Autodesk Inventor part; units mm, degrees
ref_plane "YZ Plane" through (0, 0, 0) normal (1, 0, 0) x (0, 1, 0)
ref_plane "XZ Plane" through (0, 0, 0) normal (0, 1, 0) x (-1, 0, 0)
ref_plane "XY Plane" through (0, 0, 0) normal (0, 0, 1) x (1, 0, 0)
sketch "Sketch1" plane through (0, 0, 0) normal (0, 1, 0) x (-1, 0, 0)
  line L0 (0.53, 20.25) -> (-28.77, 20.25)
  line L1 (-28.77, 20.25) -> (-28.77, -20.25)
  line L2 (-28.77, -20.25) -> (0.53, -20.25)
  line L3 (0.53, -20.25) -> (0.53, 20.25)
  point P0 (0, 0)
  dimension "d0" = 40.5
  dimension "d1" = 29.3
  dimension "d2" = -0.53
  dimension "d3" = 20.25
extrude "Plate1" add sketch "Sketch1" along normal blind 1.5
sketch "Sketch2" plane through (28.77, 0, 21.75) normal (0, 0, -1) x (-1, 0, 0)
  line L0 (29.3, 0) -> (0, 0)
  line L1 (0, 0) -> (0, 28.14)
  line L2 (0, 28.14) -> (29.3, 28.14)
  line L3 (29.3, 28.14) -> (29.3, 0)
edge flange "Flange1" height 28.14 angle 90 thickness 1.5 bend radius 0.31 thickness toward (0, 0, -1) relief tear relief width 1.5 relief depth 0.75 corner gap 0.31 corner form 0 edges at (14.12, 1.5, 20.25) (14.12, 1.5, -20.25) wall of the first edge with corners at (-0.53, 0, 21.75) (28.77, 0, 21.75) (28.77, 28.14, 21.75) (-0.53, 28.14, 21.75)
bend "Bend1"
corner "Corner1"
sketch "Sketch6" plane through (-0.53, 28.14, 21.75) normal (0, 0, 1) x (1, 0, 0)
  point P0 (0.53, -28.14)
sketch "Sketch8" plane through (28.77, 28.14, -21.75) normal (0, 0, -1) x (-1, 0, 0)
  circle A0 centre (2.5, -2.545) radius 0.7835
  circle A1 centre (2.5, -17.595) radius 0.7835
  circle A2 centre (17.6, -2.545) radius 0.7835
  circle A3 centre (17.6, -17.595) radius 0.7835
  circle A4 centre (37.6, -2.545) radius 0.7835
  circle A5 centre (37.6, -17.595) radius 0.7835
  point P0 (28.77, -28.14)
hole "Hole4" at (26.27, 25.595, -21.75) at (26.27, 10.545, -21.75) at (11.17, 25.595, -21.75) at (11.17, 10.545, -21.75) at (-8.83, 25.595, -21.75) at (-8.83, 10.545, -21.75) direction (0, 0, 1) diameter 2.1 depth 1.5
sketch "Sketch9" plane through (28.77, 28.14, -21.75) normal (0, 0, -1) x (-1, 0, 0)
  circle A0 centre (30.1, -10.07) radius 6
  point P0 (28.77, -28.14)
extrude "Cut2" cut sketch "Sketch9" against normal blind 1.5
sketch "Sketch10" plane through (-0.53, 28.14, 21.75) normal (0, 0, 1) x (1, 0, 0)
  point P0 (0.53, -28.14)
sketch "Sketch11" plane through (-0.53, 28.14, 21.75) normal (0, 0, 1) x (1, 0, 0)
  point P0 (0.53, -28.14)
sketch "Sketch15" plane through (0, 0, 0) normal (0, -1, 0) x (1, 0, 0)
  point P0 (0, 0)
sketch "Sketch16" plane through (0, 0, 0) normal (0, -1, 0) x (1, 0, 0)
  circle A0 centre (6.47, 14.94) radius 1.55
  line L0 (28.77, 19.94) -> (-0.53, 19.94)
  line L1 (-0.53, -19.94) -> (-0.53, 19.94)
  circle A1 centre (21.77, 14.94) radius 1.55
  line L2 (28.77, 19.94) -> (28.77, -19.94)
  circle A2 centre (6.47, 4.8) radius 1.55
  circle A3 centre (21.77, 4.8) radius 1.55
  point P0 (0, 0)
  dimension "d65" = 3.1
  dimension "d66" = 5
  dimension "d67" = 7
  dimension "d68" = 3.1
  dimension "d69" = 5
  dimension "d70" = 7
  dimension "d71" = 3.1
  dimension "d72" = 15.14
  dimension "d73" = 7
  dimension "d74" = 3.1
  dimension "d75" = 15.14
  dimension "d76" = 7
extrude "Cut6" cut sketch "Sketch16" against normal blind 1.5
sketch "Sketch18" plane through (-0.53, 28.14, 21.75) normal (0, 0, 1) x (1, 0, 0)
  circle A0 centre (-0.8, -10.07) radius 6
  point P0 (0.53, -28.14)
extrude "Cut7" cut sketch "Sketch18" against normal blind 1.5
fillet "Corner Round1" radius 1 4 edges at (-0.53, 28.14, -21) (28.77, 28.14, -21) (28.77, 28.14, 21) (-0.53, 28.14, 21)
sketch "Sketch19" plane through (-0.53, 1.81, 21.75) normal (0, 0, 1) x (1, 0, 0)
  circle A0 centre (6.1, 24.26) radius 0.7835
  circle A1 centre (19.32, 23.26) radius 0.7835
  circle A2 centre (26.62, 16.26) radius 0.7835
  circle A3 centre (19.32, 9.26) radius 0.7835
  circle A4 centre (6.1, 8.26) radius 0.7835
  point P0 (0.53, -1.81)
hole "Hole6" at (5.57, 26.07, 21.75) at (18.79, 25.07, 21.75) at (26.09, 18.07, 21.75) at (18.79, 11.07, 21.75) at (5.57, 10.07, 21.75) direction (0, 0, -1) diameter 2.1 depth 1.5
equation "\"d55\" = Thickness"
equation "\"d57\" = Thickness"
equation "\"d77\" = Thickness"
equation "\"d86\" = Thickness"
equation "\"d94\" = Thickness"
equation "\"d4\" = Thickness"
equation "\"d5\" = BendReliefWidth"
equation "\"d6\" = BendReliefDepth"
equation "\"d7\" = MinimumRemnant"
equation "\"d8\" = TransitionRadius"
equation "\"d11\" = BendRadius"
equation "\"d12\" = CornerReliefSize"
equation "\"d13\" = GapSize"
equation "\"d14\" = JacobiRadiusSize"
equation "\"BendReliefWidth\" = Thickness"
equation "\"BendReliefDepth\" = 0.5 * Thickness"
equation "\"CornerReliefSize\" = 4 * Thickness"
equation "\"MinimumRemnant\" = 2 * Thickness"
equation "\"TransitionRadius\" = BendRadius"
equation "\"JacobiRadiusSize\" = BendRadius"
equation "\"GapSize\" = Thickness"
properties part number "axis_25_bottom_frame" material "Aluminum 6061-AHC"
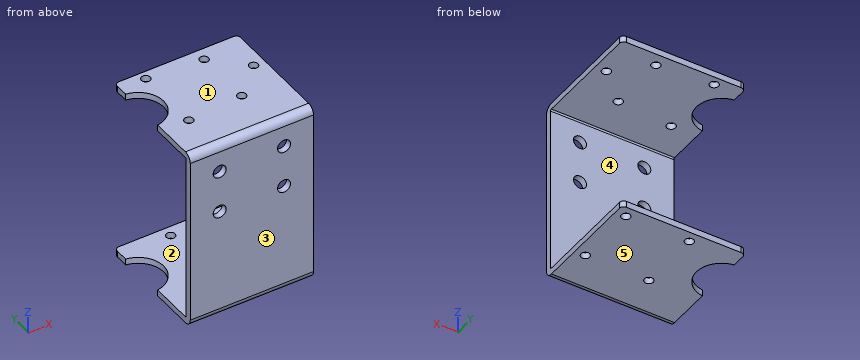
Work out the finished part from the listing and answer in its coordinate system (mm). Face numbers are marked on the shaded views. A direction names the side the tool comes from. Give positions to 0.01 mm unless a question says otherwise; leave off trailing zeros. Write each loop counter-clockwise with the first axis right and the second up, starting at its lowest first coordinate (ties: lowest second). Pieces come first, ordered by that corner, then holes. Notation, with made-up numbers: M 5,32.5 L 30,32.5 A19 cw 30,38.5 Z; hole C 30.5,75.25 d10. An arc over 180 degrees is marked long. Answer as CSV lines item,"result".
Q1. Given P1, Ø14.5, axis at x = 19.5, z = 6.5, coming from the +Y side; P2, Ø1.3, axis at x = 26.09, y = 18.07, coming from the +Z side, each flat-ended and moving along its own axis, determine where each tip first touches the part or whether it passes through.
A:
P1,"stops at y = 1.5"
P2,"stops at z = -20.25"
Q2. The mould has two halves that part along Z. Classify the marked faces 3, 4 and 5: +Z half, -Z half, draft (parallel to the pull), parting line (faces both ways), or undercut.
A:
face 3,"draft"
face 4,"undercut"
face 5,"-Z half"
Q3. A tool of negligible diameter and unlimited length cuts with its end or side. For the marked faces 1 and 2, from which of +Z, -Z, +X, -X, +Y, -Y can it reach the whole face along a straight path? Write none if from no direction.
A:
face 1,"+Z, +X, -X, +Y, -Y"
face 2,"+X, -X, +Y"
Q4. Find the intervals of material crossed by probe 1 along Y at (x, z) = (18.79, 21.15); probe 2 along Z at (x, y) = (17.75, 13.5); probe 3 along Z at (x, y) = (6.47, 0.55), in increasing order. Write a range as [from, to].
A:
probe 1,"y = [0.46, 10.02], [12.12, 24.02], [26.12, 28.14]"
probe 2,"z = [-21.75, -20.25], [20.25, 21.75]"
probe 3,"z = [-21.24, 3.25], [6.35, 13.39], [16.49, 21.24]"
Q5. A cutting plane is placed at C-C on y = 6.5. Write down the section's boundary in (x, z).
A:
outline,"M -0.53,-21.75 L 28.77,-21.75 L 28.77,-20.25 L -0.53,-20.25 Z; M -0.53,20.25 L 28.77,20.25 L 28.77,21.75 L -0.53,21.75 Z"
Q6. A cutting plane is placed at A-A on x = 18.79. Write down the section's boundary in (y, z), plus the area to 3 significant figures.
A:
outline,"M 0,-19.94 A1.81 ccw 1.81,-21.75 L 28.14,-21.75 L 28.14,-20.25 L 1.81,-20.25 A0.31 cw 1.5,-19.94 L 1.5,19.94 A0.31 cw 1.81,20.25 L 10.02,20.25 L 10.02,21.75 L 1.81,21.75 A1.81 ccw 0,19.94 Z; M 12.12,20.25 L 24.02,20.25 L 24.02,21.75 L 12.12,21.75 Z; M 26.12,20.25 L 28.14,20.25 L 28.14,21.75 L 26.12,21.75 Z"
area,"138 mm²"
Q7. A cutting plane is placed at B-B on z = 4.8. Write down the section's boundary in (x, y).
A:
outline,"M -0.53,0 L 4.92,0 L 4.92,1.5 L -0.53,1.5 Z; M 8.02,0 L 20.22,0 L 20.22,1.5 L 8.02,1.5 Z; M 23.32,0 L 28.77,0 L 28.77,1.5 L 23.32,1.5 Z"
Q8. A cutting plane is placed at D-D on x = 5.57. Write down the section's boundary in (y, z), plus the area to 3 significant figures.
A:
outline,"M 0,-19.94 A1.81 ccw 1.81,-21.75 L 28.14,-21.75 L 28.14,-20.25 L 1.81,-20.25 A0.31 cw 1.5,-19.94 L 1.5,3.54 L 0,3.54 Z; M 0,6.06 L 1.5,6.06 L 1.5,13.68 L 0,13.68 Z; M 0,16.2 L 1.5,16.2 L 1.5,19.94 A0.31 cw 1.81,20.25 L 9.02,20.25 L 9.02,21.75 L 1.81,21.75 A1.81 ccw 0,19.94 Z; M 11.12,20.25 L 25.02,20.25 L 25.02,21.75 L 11.12,21.75 Z; M 27.12,20.25 L 28.14,20.25 L 28.14,21.75 L 27.12,21.75 Z"
area,"130 mm²"
